Check sheet for the modelled part. Datum: model origin and axes. Units: mm. Face numbers are marked on the shaded views. Give positions to 0.01 mm unless a question says otherwise; leave off trailing zeros. Order: outer loops, then holes, each group sorted by start corner. A loop starts at its lowest first (then second) coordinate and runs counter-clockwise, first axis right, second up.
Item 1: Release check for a two-part mould opening along Y. For the marked faces 1, 2 and 3 record: released by +Y, released by -Y, zero draft, split by the parting line, or undercut.
Item 2: Sectioned sample at D-D on y = 16.5. Record the boundary of the cut face in (x, z), and give its area (3 significant figures).
Item 3: Sectioned sample at B-B on y = 7. Record the boundary of the cut face in (x, z).
Item 4: Gauge pin test, flat ends, axial feed: P1, Ø2.5, axis at x = 24.5, y = 31, coming from the +Z side; P2, Ø6.5, axis at x = 21.83, y = 26.45, coming from the +Z side; P3, Ø9.5, axis at x = 18.5, y = 8.5, coming from the +Z side. Record the tip position at first contact, or that the pin passes through.
Item 5: Sectioned sample at A-A on z = 16.5. Count the separate pieces of the cut face and the enclosed holes in it, and give its area (3 significant figures).
Item 6: Material ranges on line 1 along X through (y, z) = (14, 26); line 2 along X through (y, z) = (5, 40.5); line 3 along Y through (x, z) = (7, 23), recorded low to high.
Item 7: Sectioned sample at C-C on z = -2. Record the boundary of the cut face in (x, y).
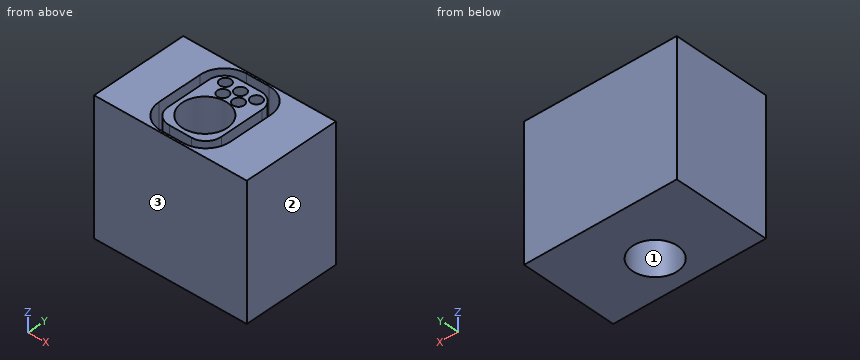
Solid Edge part; units mm, degrees
sketch "Sketch1" plane through (0, 0, 0) normal (0, 0, 1) x (1, 0, 0)
  line L0 (30.3251, 8.7316) -> (30.3251, 28.7316)
  arc A0 (30.3251, 28.7316) -> (23.3251, 35.7316) centre (23.3251, 28.7316) ccw
  line L1 (23.3251, 35.7316) -> (13.3251, 35.7316)
  arc A1 (13.3251, 35.7316) -> (6.3251, 28.7316) centre (13.3251, 28.7316) ccw
  line L2 (6.3251, 28.7316) -> (6.3251, 8.7316)
  arc A2 (6.3251, 8.7316) -> (13.3251, 1.7316) centre (13.3251, 8.7316) ccw
  line L3 (13.3251, 1.7316) -> (23.3251, 1.7316)
  arc A3 (23.3251, 1.7316) -> (30.3251, 8.7316) centre (23.3251, 8.7316) ccw
  line L4 (52.6751, 40.5816) -> (-16.0249, 40.5816)
  line L5 (-16.0249, 40.5816) -> (-16.0249, -3.1184)
  line L6 (-16.0249, -3.1184) -> (52.6751, -3.1184)
  line L7 (52.6751, -3.1184) -> (52.6751, 40.5816)
  circle A4 centre (14.8251, 26.4516) radius 2.5
  circle A5 centre (25.3251, 31.4516) radius 2.5
  circle A6 centre (21.8251, 26.4516) radius 2.5
  circle A7 centre (18.3562, 13.7016) radius 10.15
  line L8 (18.3251, 23.8516) -> (18.3251, 23.8515) construction
  line L9 (18.3562, 23.8516) -> (18.3251, 23.8516) construction
  circle A8 centre (18.3535, 31.217) radius 2.5
  circle A9 centre (11.3251, 31.4516) radius 2.5
  line L10 (23.3251, 39.7316) -> (13.3251, 39.7316)
  arc A10 (13.3251, 39.7316) -> (2.3251, 28.7316) centre (13.3251, 28.7316) ccw
  line L11 (2.3251, 28.7316) -> (2.3251, 8.7316)
  arc A11 (2.3251, 8.7316) -> (13.3251, -2.2684) centre (13.3251, 8.7316) ccw
  line L12 (13.3251, -2.2684) -> (23.3251, -2.2684)
  arc A12 (23.3251, -2.2684) -> (34.3251, 8.7316) centre (23.3251, 8.7316) ccw
  line L13 (34.3251, 8.7316) -> (34.3251, 28.7316)
  arc A13 (34.3251, 28.7316) -> (23.3251, 39.7316) centre (23.3251, 28.7316) ccw
extrude "Protrusion1" add sketch "Sketch1" along normal blind 50
sketch "Sketch2" plane through (0, 0, 0) normal (0, 0, 1) x (1, 0, 0)
  line L0 (52.6751, 40.5816) -> (-16.0249, 40.5816)
  line L1 (-16.0249, 40.5816) -> (-16.0249, -3.1184)
  line L2 (-16.0249, -3.1184) -> (52.6751, -3.1184)
  line L3 (52.6751, -3.1184) -> (52.6751, 40.5816)
extrude "Protrusion2" add sketch "Sketch2" against normal blind 10
sketch "Sketch3" plane through (18.3562, 13.7016, 0) normal (0, 0, 1) x (0, -1, 0)
  circle A0 centre (0, 0) radius 10.15
extrude "Cutout1" cut sketch "Sketch3" against normal blind 780
Report:
1. face 1: undercut
1. face 2: zero draft
1. face 3: released by -Y
2. outline: (-16.02, -10) - (8.6, -10) - (8.6, 50) - (6.33, 50) - (6.33, 0) - (2.33, 0) - (2.33, 50) - (-16.02, 50) - close; (28.11, -10) - (52.68, -10) - (52.68, 50) - (34.33, 50) - (34.33, 0) - (30.33, 0) - (30.33, 50) - (28.11, 50) - close
2. area: 2,550 mm2
3. outline: (-16.02, -10) - (10.73, -10) - (10.73, 50) - (6.54, 50) - (6.54, 0) - (2.46, 0) - (2.46, 50) - (-16.02, 50) - close; (25.98, -10) - (52.68, -10) - (52.68, 50) - (34.19, 50) - (34.19, 0) - (30.11, 0) - (30.11, 50) - (25.98, 50) - close
4. P1: stops at z = 0
4. P2: stops at z = 50
4. P3: passes through
5. separate pieces: 2
5. enclosed holes: 7
5. area: 2,110 mm2
6. line 1: x = -16.02 to 2.33, 6.33 to 8.21, 28.5 to 30.33, 34.33 to 52.68
6. line 2: x = -16.02 to 2.98, 7.4 to 13.13, 23.58 to 29.25, 33.67 to 52.68
6. line 3: y = -3.12 to -0.27, 5.73 to 31.73, 37.73 to 40.58
7. outline: (-16.02, -3.12) - (52.68, -3.12) - (52.68, 40.58) - (-16.02, 40.58) - close; hole circle Ø20.3 at (18.36, 13.7)
